from build123d import *

# Parameters (mm, degrees)
F1_DEPTH       = 30.48
F4_D           = 13.97
F4_DEPTH       = 19.051
F4_ON_F2_D     = 13.97
F4_ON_F2_DEPTH = 19.051
F6_D           = 3.175
F8_SIZE        = 5.08
F9_SIZE        = 6.34999
F10_D          = 4.445
F10_DEPTH      = 12.7
F10_TIP        = 1.3354127258
F12_D          = 4.445
F12_DEPTH      = 12.7
F12_TIP        = 1.3354127258
F13_R          = 12.7


# Not quite as in the source:
# - a fillet or chamfer is up to 0.001 mm smaller than in the source, because OpenCascade refuses the exact size
# - a feature names something its author has since deleted; it is built from what else it names


with BuildPart() as f1:
    # F0 (on Top) → F1 (new body)
    with BuildSketch(Plane.XY):
        Polygon((38.1, 57.15), (-50.8, 57.15), (-50.8, -12.7), (-31.75, -12.7), (-31.75, 12.7), (-38.1, 12.7), (-38.1, 38.1), (25.4, 38.1), (25.4, 12.7), (19.05, 12.7), (19.05, -12.7), (38.1, -12.7), align=None)
    extrude(amount=F1_DEPTH)

    # F4 (through all, one way)
    with BuildSketch(Plane(origin=(19.05, 0, 0), x_dir=(0, -1, 0), z_dir=(-1, 0, 0))):
        with Locations((0, 15.24)):
            Circle(F4_D / 2)
    extrude(amount=-F4_DEPTH, mode=Mode.SUBTRACT)

    # F4 on F2 (through all, one way)
    with BuildSketch(Plane.YZ.offset(-31.75)):
        with Locations((0, 15.24)):
            Circle(F4_ON_F2_D / 2)
    extrude(amount=-F4_ON_F2_DEPTH, mode=Mode.SUBTRACT)

    # F6 (through all)
    with Locations(Plane(origin=(-50.8, 0, 0), x_dir=(0, -1, 0), z_dir=(-1, 0, 0))):
        with Locations((-6.706288951, 22.003272388), (6.4929844043, 22.2083615897), (6.706288951, 8.476727612), (-6.706288951, 8.476727612)):
            Hole(F6_D / 2)

    # F8
    f8_edges = [f1.edges().sort_by_distance(p)[0] for p in [
        (-38.1, 38.1, 15.24),
        (25.4, 38.1, 15.24),
    ]]
    chamfer(f8_edges, length=F8_SIZE)

    # F9 (size 6.35 in the source; OpenCascade refuses exactly that, so slightly less here)
    f9_edges = [f1.edges().sort_by_distance(p)[0] for p in [
        (25.4, 12.7, 15.24),
        (-38.1, 12.7, 15.24),
    ]]
    chamfer(f9_edges, length=F9_SIZE)

    # F10
    with Locations(Plane(origin=(-50.8, 0, 0), x_dir=(0, -1, 0), z_dir=(-1, 0, 0))):
        with Locations((6.4929844043, 22.2083615897), (6.706288951, 8.476727612), (-6.706288951, 8.476727612), (-6.706288951, 22.003272388)):
            Hole(F10_D / 2, depth=F10_DEPTH)
            with Locations((0, 0, -(F10_DEPTH + F10_TIP / 2))):  # 118° drill point
                Cone(0, F10_D / 2, F10_TIP, mode=Mode.SUBTRACT)

    # F12
    with Locations(Plane.YZ.offset(38.1)):
        with Locations((-6.706288951, 8.476727612), (-6.4929844043, 22.2083615897), (6.706288951, 22.003272388), (6.706288951, 8.476727612)):
            Hole(F12_D / 2, depth=F12_DEPTH)
            with Locations((0, 0, -(F12_DEPTH + F12_TIP / 2))):  # 118° drill point
                Cone(0, F12_D / 2, F12_TIP, mode=Mode.SUBTRACT)

    # F13
    f13_edges = [f1.edges().sort_by_distance(p)[0] for p in [
        (-41.275, -12.7, 30.48),
        (28.575, -12.7, 30.48),
        (28.575, -12.7, 0),
        (-41.275, -12.7, 0),
    ]]
    fillet(f13_edges, radius=F13_R)


solid = f1.part
Geometry check sheet. Reference: the model listing, model coordinates, mm. A direction names the side the tool comes from. Coordinates: 2 decimals unless noted, no trailing zeros. Order: outer loops, then holes, each group sorted by start corner. A loop starts at its lowest first (then second) coordinate and runs counter-clockwise, first axis right, second up. Notation, with made-up numbers: (-12, 87.25) - (-7, 87.25) arc R31 cw to (-7, 113.25) - close; hole circle Ø10 at (16.25, 33). An arc over 180 degrees is marked (long way). Answer in a Markdown table with one row per item. Add a question column.
1) Release check for a two-part mould opening along Z. For faces 1 (the flat face through (-41, -12.7, 15)), 2 (the cylindrical face through (-34.69, 7.44, 7.07)), 3 (the cylindrical face through (31.66, 7, 10.68)) record: +Z half, -Z half, draft (parallel to the pull), parting line (faces both ways), or undercut.
2) Cross-section at A-A, the plane y = 2.5. Record the cut outline in (x, z).
3) Cross-section at C-C, the plane x = -18. Record the cut outline in (y, z).
4) Material ranges on line 1 along X through (y, z) = (27.5, 4.5); line 2 along Y through (x, z) = (-40.5, 15.5); line 3 along X through (y, z) = (12.5, 2), recorded low to high. Write a range as [from, to].
5) Gauge pin test, flat ends, axial feed: P1, Ø3.5, axis at y = -6.49, z = 22.21, coming from the -X side; P2, Ø4, axis at y = 6.71, z = 8.48, coming from the -X side; P3, Ø16, axis at y = 0, z = 15.24, coming from the +X side; P4, Ø3.5, axis at y = 6.71, z = 8.48, coming from the +X side. Record the tip position at first contact, or that the pin passes through.
6) Set-up check for faces 4 (the cylindrical face through (31.66, -6.2, 24.41)), 5 (the flat face through (-35.52, 35.6, 15.03)), 6 (the flat face through (-6, 57.15, 15)): record each of +Z, -Z, +X, -X, +Y, -Y from which the full face is reachable in a straight line by a thin tool's end or side.
Check result:
| question | item | result |
|---|---|---|
| 1 | face 1 | draft |
| 1 | face 2 | undercut |
| 1 | face 3 | undercut |
| 2 | outline | (-50.8, 0) - (-31.75, 0) - (-31.75, 8.72) - (-50.8, 8.72) - close; (-50.8, 21.76) - (-31.75, 21.76) - (-31.75, 30.48) - (-50.8, 30.48) - close; (19.05, 0) - (38.1, 0) - (38.1, 8.72) - (19.05, 8.72) - close; (19.05, 21.76) - (38.1, 21.76) - (38.1, 30.48) - (19.05, 30.48) - close |
| 3 | outline | (38.1, 0) - (57.15, 0) - (57.15, 30.48) - (38.1, 30.48) - close |
| 4 | line 1 | x = [-50.8, -38.1], [25.4, 38.1] |
| 4 | line 2 | y = [-12.7, -6.98], [6.98, 57.15] |
| 4 | line 3 | x = [-50.8, -31.75], [19.05, 38.1] |
| 5 | P1 | stops at x = -37.82 |
| 5 | P2 | stops at x = -37.97 |
| 5 | P3 | stops at x = 38.1 |
| 5 | P4 | stops at x = 25.12 |
| 6 | face 4 | +X |
| 6 | face 5 | +Z, -Z |
| 6 | face 6 | +Z, -Z, +X, -X, +Y |
